from build123d import *

# Parameters (mm, degrees)
SKETCH1_W           = 21
SKETCH1_H           = 21
BOSS_EXTRUDE1_DEPTH = 114
SKETCH3_R           = 2.5
CUT_EXTRUDE1_DEPTH  = 117.392654407
SKETCH4_R           = 2.5
CUT_EXTRUDE2_DEPTH  = 117.392654407


with BuildPart() as part:
    # Sketch1 → Boss-Extrude1 (new body)
    with BuildSketch(Plane(origin=(0, 0, 0), x_dir=(1, 0, 0), z_dir=(0, 1, 0))):
        Rectangle(SKETCH1_W, SKETCH1_H)
    extrude(amount=BOSS_EXTRUDE1_DEPTH)

    # Sketch3 → Cut-Extrude1 (cut, through all)
    with BuildSketch(Plane.XY.offset(10.5)):
        with Locations((0, 99)):
            Circle(SKETCH3_R)
        with Locations((0, 25)):
            Circle(SKETCH3_R)
    extrude(amount=-CUT_EXTRUDE1_DEPTH, mode=Mode.SUBTRACT)

    # Sketch4 → Cut-Extrude2 (cut, through all)
    with BuildSketch(Plane(origin=(10.5, 0, 0), x_dir=(0, 0, -1), z_dir=(1, 0, 0))):
        with Locations((0, 89)):
            Circle(SKETCH4_R)
        with Locations((0, 15)):
            Circle(SKETCH4_R)
    extrude(amount=-CUT_EXTRUDE2_DEPTH, mode=Mode.SUBTRACT)


solid = part.part
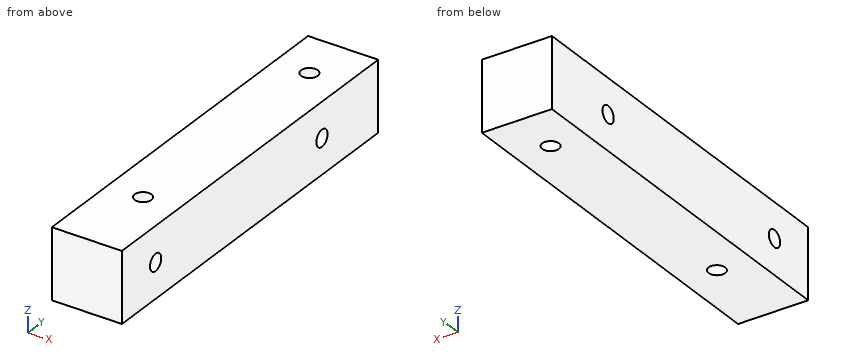
Here's how the part is built. I have some questions about the finished solid (model axes, mm). Coordinates: 2 decimals unless noted, no trailing zeros. Write each loop counter-clockwise with the first axis right and the second up, starting at its lowest first coordinate (ties: lowest second). Pieces come first, ordered by that corner, then holes. Notation, with made-up numbers: (26, -22.5) - (84, -22.5) arc R22 cw to (84, 1.5) - close; hole circle Ø6 at (-10, 21). An arc over 180 degrees is marked (long way). Use one line per item in the form item = value.
1) Suppose I cut it at B-B, the plane x = 0. Write out the boundary of the cut face in (y, z), plus the area to 3 significant figures.
Solved:
outline = (0, -10.5) - (22.5, -10.5) - (22.5, 10.5) - (0, 10.5) - close; (27.5, -10.5) - (96.5, -10.5) - (96.5, 10.5) - (27.5, 10.5) - close; (101.5, -10.5) - (114, -10.5) - (114, 10.5) - (101.5, 10.5) - close; hole circle Ø5 at (15, 0); hole circle Ø5 at (89, 0)
area = 2,140 mm2
2) Suppose I cut it at C-C, the plane y = 25. Write out the boundary of the cut face in (x, z).
Solved:
outline = (-10.5, -10.5) - (-2.5, -10.5) - (-2.5, 10.5) - (-10.5, 10.5) - close; (2.5, -10.5) - (10.5, -10.5) - (10.5, 10.5) - (2.5, 10.5) - close
3) Suppose I cut it at A-A, the plane z = 0. Write out the boundary of the cut face in (x, y), plus the area to 3 significant figures.
Solved:
outline = (-10.5, 0) - (10.5, 0) - (10.5, 12.5) - (-10.5, 12.5) - close; (-10.5, 17.5) - (10.5, 17.5) - (10.5, 86.5) - (-10.5, 86.5) - close; (-10.5, 91.5) - (10.5, 91.5) - (10.5, 114) - (-10.5, 114) - close; hole circle Ø5 at (0, 25); hole circle Ø5 at (0, 99)
area = 2,140 mm2
4) I need wall thicknesses on line 1 (Y direction, x = 5.5, z = 0); line 2 (Y direction, x = 0, z = -4.25); line 3 (Y direction, x = -1.25, z = 2.25). Which ranges of each line are inside material? Lowest first, please.
Solved:
line_1 = 0 to 12.5, 17.5 to 86.5, 91.5 to 114
line_2 = 0 to 22.5, 27.5 to 96.5, 101.5 to 114
line_3 = 0 to 13.91, 16.09 to 22.83, 27.17 to 87.91, 90.09 to 96.83, 101.17 to 114
